Study the drawing (mm; zero at the part's minimum x, y, z) and answer. Give positions to 0.01 mm unless a question says otherwise; leave off trailing zeros. Loops run counter-clockwise (first coordinate to the right, second up) from the corner with the lowest first, then second, coordinate; pieces in that order, holes last. Notation, with made-up numbers: (62.25, 48) - (106.25, 48) arc R25 cw to (106.25, 86) - close; hole circle Ø8 at (74, 21). An arc over 180 degrees is marked (long way). Use one line per item in the form item = value. Start each with the question number.
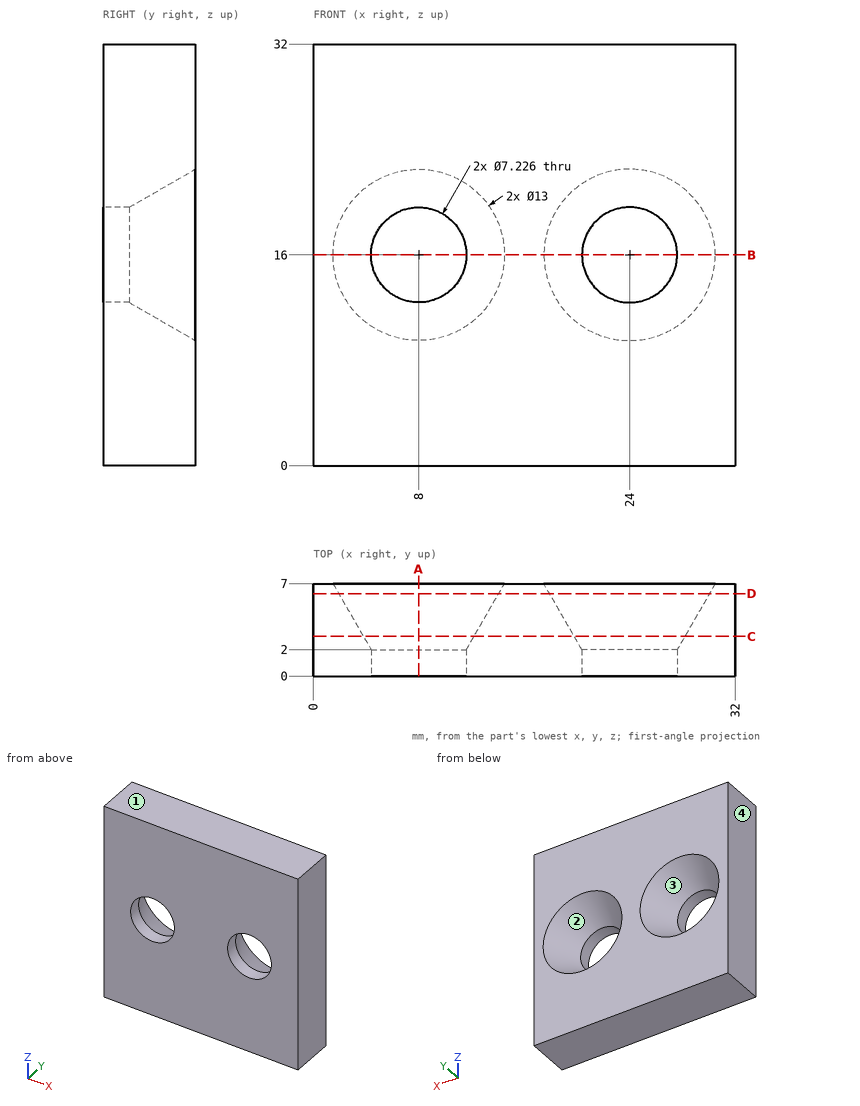
1) Find the intervals of material crossed by probe 1 along Z at (x, y) = (24, 1.3); probe 2 along X at (y, z) = (6.5, 11) (1 decimal); probe 3 along X at (y, z) = (4, 16.5), in increasing order.
2) Determine the mould class of the marked faces 1, 2, 3 and 4 for opening direction X: released by +X, released by -X, zero draft, split by the parting line, or undercut.
3) A cutting plane is placed at B-B (z = 16). Give the vertices of the cut face in (x, y).
4) A cutting plane is placed at D-D (y = 6.25). Give the vertices of the cut face in (x, z), plus the area to 3 significant figures.
5) A cutting plane is placed at A-A (x = 8). Give the vertices of the cut face in (y, z).
6) Flat-ended cylindrical pins translate along their axes: pin 1 Ø6 at (x, z) = (15.5, 9) entering from -Y; pin 2 Ø6.5 at (x, z) = (8, 16) entering from -Y; pin 3 Ø9.5 at (x, z) = (24, 16) entering from +Y. Find the tip coordinate at first contact, or state that the pin passes through.
7) A cutting plane is placed at C-C (y = 3). Give the vertices of the cut face in (x, z).
Answer sheet:
q1.probe_1 = 0 to 12.39, 19.61 to 32
q1.probe_2 = 0 to 4.3, 11.7 to 20.3, 27.7 to 32
q1.probe_3 = 0 to 3.26, 12.74 to 19.26, 28.74 to 32
q2.face_1 = zero draft
q2.face_2 = undercut
q2.face_3 = undercut
q2.face_4 = released by -X
q3.outline = (0, 0) - (4.39, 0) - (4.39, 2) - (1.5, 7) - (0, 7) - close; (11.61, 0) - (20.39, 0) - (20.39, 2) - (17.5, 7) - (14.5, 7) - (11.61, 2) - close; (27.61, 0) - (32, 0) - (32, 7) - (30.5, 7) - (27.61, 2) - close
q4.outline = (0, 0) - (32, 0) - (32, 32) - (0, 32) - close; hole circle Ø12.13 at (8, 16); hole circle Ø12.13 at (24, 16)
q4.area = 793 mm²
q5.outline = (0, 0) - (7, 0) - (7, 9.5) - (2, 12.39) - (0, 12.39) - close; (0, 19.61) - (2, 19.61) - (7, 22.5) - (7, 32) - (0, 32) - close
q6.pin_1 = 0
q6.pin_2 = through
q6.pin_3 = 3.97
q7.outline = (0, 0) - (32, 0) - (32, 32) - (0, 32) - close; hole circle Ø8.38 at (8, 16); hole circle Ø8.38 at (24, 16)
